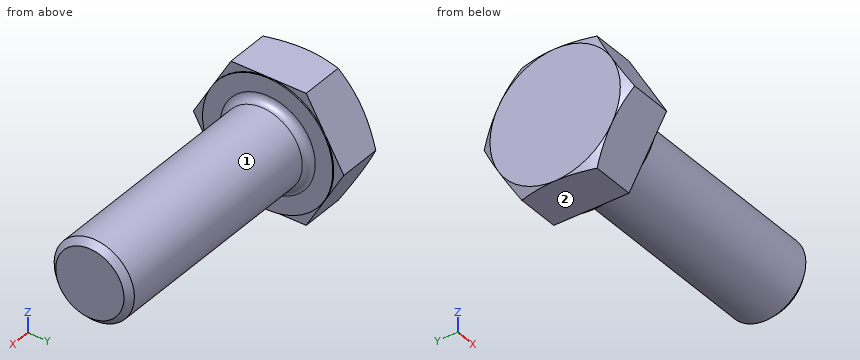
```python
from build123d import *

# Parameters (mm, degrees)
BASEHEAD_DEPTH = 15.9258
SKETCH4_W      = 0.381
SKETCH4_H      = 28.592632361
HEADFILLET_R   = 2.3622


with BuildPart() as part:
    # Sketch1 → BaseHead (new body)
    with BuildSketch(Plane(origin=(0, 0, 0), x_dir=(0, 0, -1), z_dir=(1, 0, 0))):
        Polygon((20.6375, 11.91506618), (20.6375, -11.91506618), (0, -23.830132361), (-20.6375, -11.91506618), (-20.6375, 11.91506618), (0, 23.830132361), align=None)
    extrude(amount=BASEHEAD_DEPTH)

    # BodySke → BaseBody (revolve)
    with BuildSketch(Plane.XY, mode=Mode.PRIVATE) as basebody_sk:
        Polygon((0, 0), (92.1258, 0), (92.1258, 10.8077), (90.2335, 12.7), (0, 12.7), align=None)
    revolve(basebody_sk.sketch.rotate(Axis((0, 0, 0), (1, 0, 0)), 90), axis=Axis((0, 0, 0), (1, 0, 0)))

    # Sketch3 → HeadChamfer (revolve, cut)
    with BuildSketch(Plane.XY):
        Polygon((0, 20.6375), (5.509441362, 30.180132361), (5.509441362, 36.530132361), (-12.7, 36.530132361), (-12.7, 20.6375), align=None)
    revolve(axis=Axis((0, 0, 0), (1, 0, 0)), mode=Mode.SUBTRACT)

    # Sketch4 → BearingFace (revolve, cut)
    with BuildSketch(Plane.XY, mode=Mode.PRIVATE) as bearingface_sk:
        with Locations((15.7353, 34.933816181)):
            Rectangle(SKETCH4_W, SKETCH4_H)
    revolve(bearingface_sk.sketch.rotate(Axis((0, 0, 0), (1, 0, 0)), 270), axis=Axis((0, 0, 0), (1, 0, 0)), mode=Mode.SUBTRACT)

    # HeadFillet
    headfillet_edges = [part.edges().sort_by_distance(p)[0] for p in [
        (15.9258, 0, -12.7),
    ]]
    fillet(headfillet_edges, radius=HEADFILLET_R)


solid = part.part
```
Geometry check sheet. Reference: the model listing, model coordinates, mm. Face numbers are marked on the shaded views. A direction names the side the tool comes from. Coordinates: 2 decimals unless noted, no trailing zeros. Loops run counter-clockwise (first coordinate to the right, second up) from the corner with the lowest first, then second, coordinate; pieces in that order, holes last.
Item 1: Thickness scan on line 1 (Z direction, x = 7, y = 16.5); line 2 (X direction, y = -1, z = 17); line 3 (Z direction, x = 19, y = -7.5). Record the ranges inside material, lowest first.
Item 2: Sectioned sample at A-A, the plane x = 72. Record the boundary of the cut face in (y, z).
Item 3: Access from +Z, -Z, +X, -X, +Y, -Y to the whole of each face (thin tool, end or side, straight path). Record for the marked faces 1 and 2.
Item 4: Go/stop test with flat-tipped pins: pin 1 Ø8.5 at (y, z) = (9, -14) entering from +X; pin 2 Ø12 at (x, y) = (65.5, 6) entering from +Z; pin 3 Ø6 at (x, z) = (21.5, 5) entering from +Y. Record where each tip stops, or that it passes through.
Check result:
1. line 1: z = -12.7 to 12.7
1. line 2: x = 0 to 15.93
1. line 3: z = -10.25 to 10.25
2. outline: circle Ø25.4 at (0, 0)
3. face 1: +X
3. face 2: -Z, +X, -X, +Y, -Y
4. pin 1: stops at x = 90.54
4. pin 2: stops at z = 12.7
4. pin 3: stops at y = 12.54
